from build123d import *

# Parameters (mm, degrees)
F0_R     = 12.7
F1_DEPTH = 19.05
F2_R     = 6.35
F3_DEPTH = 12.7
F4_R     = 12.7
F5_DEPTH = 19.05
F6_R     = 2.54
F7_DEPTH = 50.8


with BuildPart() as f1:
    # F0 (on Top) → F1 (new body)
    with BuildSketch(Plane.XY):
        Circle(F0_R)
    extrude(amount=F1_DEPTH)

    # F2 (on face) → F3 (join)
    with BuildSketch(Plane.XY.offset(19.05)):
        Circle(F2_R)
    extrude(amount=F3_DEPTH)

    # F4 (on face) → F5 (join)
    with BuildSketch(Plane.XY.offset(31.75)):
        Circle(F4_R)
    extrude(amount=F5_DEPTH)

    # F6 (on face) → F7 (cut)
    with BuildSketch(Plane(origin=(0, 0, 0), x_dir=(1, 0, 0), z_dir=(0, 0, -1))):
        Circle(F6_R)
    extrude(amount=-F7_DEPTH, mode=Mode.SUBTRACT)


solid = f1.part
Check sheet for the modelled part. Datum: model origin and axes. Units: mm. A direction names the side the tool comes from. Round coordinates to 2 decimals unless told otherwise and drop trailing zeros. Write each loop counter-clockwise with the first axis right and the second up, starting at its lowest first coordinate (ties: lowest second). Pieces come first, ordered by that corner, then holes. Notation, with made-up numbers: (-1.75, 66) - (28.25, 66) arc R24 cw to (28.25, 84) - close; hole circle Ø10 at (49, 67.5). An arc over 180 degrees is marked (long way). Return JSON: item names as keys, results as strings.
Q1. Draft check along Z on faces 1 (the flat face through (3, 0, 50.8)), 2 (the flat face through (3, 6, 19.05)), 3 (the cylindrical face through (-2.75, -12.4, 9.39)). Enter one of: released by +Z, released by -Z, zero draft, split by the parting line, or undercut.
Returned:
{"face 1": "released by +Z", "face 2": "undercut", "face 3": "zero draft"}
Q2. Scan lines: L1, parallel to Y at x = 0, z = 24; L2, parallel to Z at x = 8.75, y = -4; L3, parallel to Y at x = 0, z = 15. Record each from-to range of solid material in increasing order. Write a range as from..to.
Returned:
{"L1": "y = -6.35..-2.54, 2.54..6.35", "L2": "z = 0..19.05, 31.75..50.8", "L3": "y = -12.7..-2.54, 2.54..12.7"}
Q3. Cross-section at C-C (z = 26). Record the boundary of the cut face in (x, y), then the cut area to 3 significant figures.
Returned:
{"outline": "circle Ø12.7 at (0, 0); hole circle Ø5.08 at (0, 0)", "area": "106 mm²"}
Q4. Cross-section at D-D (x = -5.75). Record the boundary of the cut face in (y, z), then the cut area to 3 significant figures.
Returned:
{"outline": "(-11.32, 0) - (11.32, 0) - (11.32, 19.05) - (2.69, 19.05) - (2.69, 31.75) - (11.32, 31.75) - (11.32, 50.8) - (-11.32, 50.8) - (-11.32, 31.75) - (-2.69, 31.75) - (-2.69, 19.05) - (-11.32, 19.05) - close", "area": "931 mm²"}
Q5. Depth check by flat-ended pin: P1, Ø2, axis at x = 6.5, z = 35.5, coming from the +Y side; P2, Ø8, axis at x = -8.5, z = 28.5, coming from the +Y side; P3, Ø1.5, axis at x = 7, z = 38, coming from the -Y side. Enter the tip coordinate at first touch or a pass-through.
Returned:
{"P1": "stops at y = 11.45", "P2": "stops at y = 11.1", "P3": "stops at y = -11.06"}
Q6. Access from +Z, -Z, +X, -X, +Y, -Y to the whole of each face (thin tool, end or side, straight path). Record for faces 4 (the flat face through (3, 0, 0)), 5 (the cylindrical face through (-1.38, -6.2, 25.31)).
Returned:
{"face 4": "-Z, +X, -X, +Y, -Y", "face 5": "none"}
Q7. Cross-section at A-A (x = 0). Record the boundary of the cut face in (y, z).
Returned:
{"outline": "(-12.7, 0) - (-2.54, 0) - (-2.54, 50.8) - (-12.7, 50.8) - (-12.7, 31.75) - (-6.35, 31.75) - (-6.35, 19.05) - (-12.7, 19.05) - close; (2.54, 0) - (12.7, 0) - (12.7, 19.05) - (6.35, 19.05) - (6.35, 31.75) - (12.7, 31.75) - (12.7, 50.8) - (2.54, 50.8) - close"}
